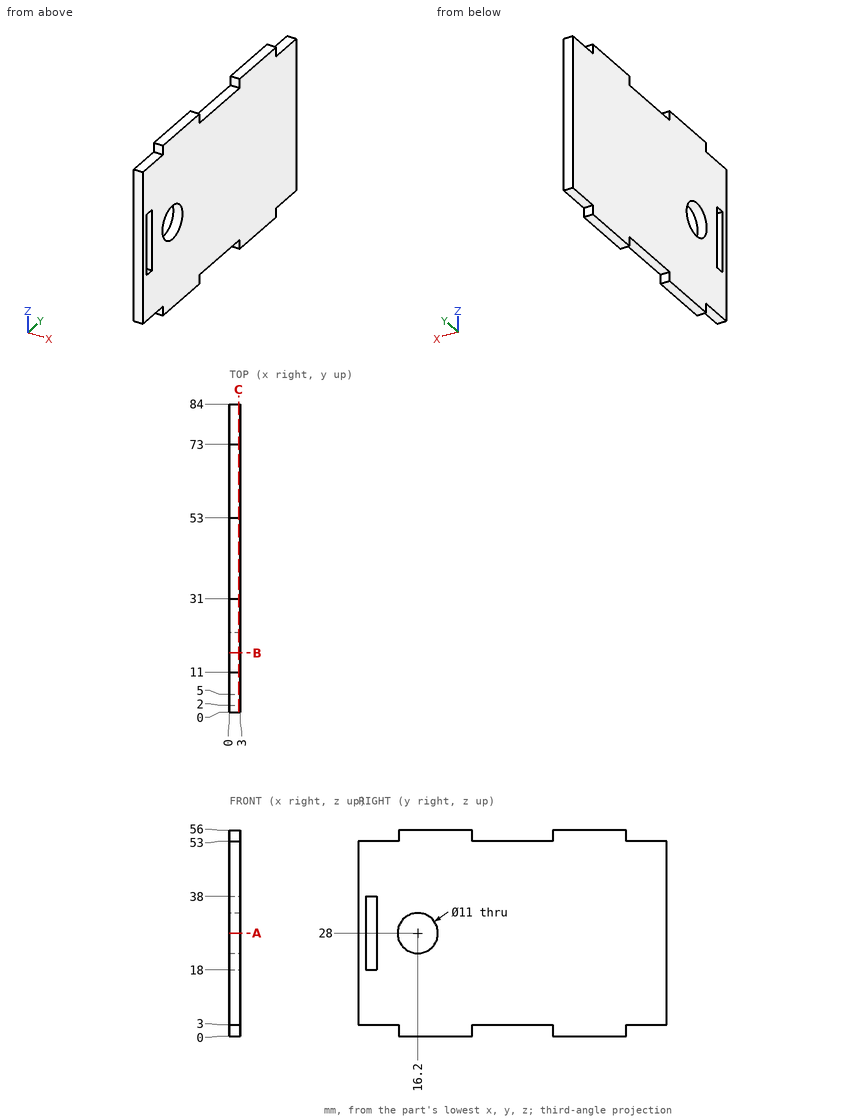
Can you work these out from the drawing? Everything is in mm from the part's minimum corner. Round coordinates to 2 decimals unless told otherwise and drop trailing zeros. Loops run counter-clockwise (first coordinate to the right, second up) from the corner with the lowest first, then second, coordinate; pieces in that order, holes last. Notation, with made-up numbers: (30.5, -40) -> (46.5, -40) arc R22 cw to (46.5, -1) -> close; hole circle Ø9 at (26.25, 23.5). An arc over 180 degrees is marked (long way). Use CSV: the item, a comma, the result in double quotes.
(1) If I drill on probe 1 along Y at (x, z) = (0.95, 28); probe 2 along Z at (x, y) = (0.65, 16.5); probe 3 along Y at (x, z) = (2.4, 30), over which ranges is the centre line in solid material (lowest first)? Write a range as [from, to].
Return value:
probe 1,"y = [0, 2], [5, 10.7], [21.7, 84]"
probe 2,"z = [0, 22.51], [33.49, 56]"
probe 3,"y = [0, 2], [5, 11.08], [21.32, 84]"
(2) Will these pins go through, and if not, where does the flat tip stop? pin 1 Ø1.5 at (x, z) = (2, 54) entering from +Y; pin 2 Ø0.9 at (x, y) = (1.5, 80) entering from +Z; pin 3 Ø1.5 at (x, y) = (1.5, 78) entering from -Z.
Return value:
pin 1,"stops at y = 73"
pin 2,"stops at z = 53"
pin 3,"stops at z = 3"
(3) Suppose I cut it at C-C on x = 2.55. Write out the boundary of the cut face in (y, z).
Return value:
outline,"(0, 3) -> (11, 3) -> (11, 0) -> (31, 0) -> (31, 3) -> (53, 3) -> (53, 0) -> (73, 0) -> (73, 3) -> (84, 3) -> (84, 53) -> (73, 53) -> (73, 56) -> (53, 56) -> (53, 53) -> (31, 53) -> (31, 56) -> (11, 56) -> (11, 53) -> (0, 53) -> close; hole (2, 18) -> (5, 18) -> (5, 38) -> (2, 38) -> close; hole circle Ø11 at (16.2, 28)"
(4) Suppose I cut it at B-B on y = 16.2. Write out the boundary of the cut face in (x, z).
Return value:
outline,"(0, 0) -> (3, 0) -> (3, 22.5) -> (0, 22.5) -> close; (0, 33.5) -> (3, 33.5) -> (3, 56) -> (0, 56) -> close"
(5) Suppose I cut it at A-A on z = 28. Write out the boundary of the cut face in (x, y), plus the area to 3 significant figures.
Return value:
outline,"(0, 0) -> (3, 0) -> (3, 2) -> (0, 2) -> close; (0, 5) -> (3, 5) -> (3, 10.7) -> (0, 10.7) -> close; (0, 21.7) -> (3, 21.7) -> (3, 84) -> (0, 84) -> close"
area,"210 mm²"
